The listing builds one solid part. Answer for the finished solid, in the listing's coordinates (mm). A direction names the side the tool comes from. Give positions to 0.01 mm unless a question says otherwise; leave off trailing zeros. Loops run counter-clockwise (first coordinate to the right, second up) from the corner with the lowest first, then second, coordinate; pieces in that order, holes last. Notation, with made-up numbers: M -35.75,15 L -25.75,15 A26 ccw -25.75,41 Z; hole C 78.25,-17 d2. An arc over 180 degrees is marked long. Return JSON: item names as keys, results as strings.
Autodesk Inventor part; units mm, degrees
ref_plane "YZ Plane" through (0, 0, 0) normal (1, 0, 0) x (0, 1, 0)
ref_plane "XZ Plane" through (0, 0, 0) normal (0, 1, 0) x (-1, 0, 0)
ref_plane "XY Plane" through (0, 0, 0) normal (0, 0, 1) x (1, 0, 0)
sketch "Эскиз1" plane through (0, 0, 0) normal (0, 0, 1) x (1, 0, 0)
  line L0 (0, 5) -> (0, 0)
  line L1 (0, 0) -> (36, 0)
  line L2 (36, 0) -> (36, 10)
  line L3 (36, 10) -> (16, 10)
  line L4 (16, 10) -> (16, 5)
  line L5 (16, 5) -> (0, 5)
  dimension "d0" = 5
  dimension "d1" = 20
  dimension "d3" = 10
  dimension "d4" = 36
revolve "Вращение1" add sketch "Эскиз1" angle 360 about axis through (0, 5, 0) along (0, -1, 0)
sketch "Эскиз2" plane through (0, 0, 0) normal (1, 0, 0) x (0, 1, 0)
  line L0 (-2, 0) -> (12, 0)
  line L1 (0, -34) -> (0, 64)
  line L2 (0, 0) -> (0, 50)
  line L3 (0, 50) -> (10, 50)
  line L4 (10, 50) -> (10, 0)
  line L5 (0, 0) -> (10, 0)
  line L6 (10, 36) -> (0, 36)
  dimension "d6" = 10
  dimension "d7" = 50
revolve "Вращение2" add sketch "Эскиз2" angle 360 about axis through (0, -10, 0) along (0, 1, 0)
chamfer "Фаска1" distance 1 angle 45 1 edges at (0, 0, -50)
sketch "Эскиз3" plane through (0, 0, 0) normal (0, -1, 0) x (1, 0, 0)
  circle A0 centre (0, 0) radius 42.5 construction
  circle A1 centre (0, 42.5) radius 5.5
  line L0 (0, -70) -> (0, 70)
  line L1 (-70, 0) -> (70, 0)
  dimension "d10" = 85
  dimension "d9" = 11
hole "Отверстие1" at (0, 0, 42.5) direction (0, 1, 0) diameter 6.2 depth 15 tip angle 118 counterbore diameter 11 counterbore depth 6.8
pattern_circular "Круговой массив1" count 6 over 360 about axis through (0, -10, 0) along (0, 1, 0) of "Отверстие1"
sketch "Эскиз4" plane through (0, 10, 0) normal (0, 1, 0) x (1, 0, 0)
  circle A0 centre (0, 0) radius 36
  circle A1 centre (0, 0) radius 16
  circle A2 centre (0, 0) radius 16
  circle A3 centre (0, 0) radius 36
  dimension "d27" = 72
extrude "Выдавливание2" add sketch "Эскиз4" along normal blind 8
fillet "Сопряжение1" radius 1.3 1 edges at (-36, 10, 0)
sketch "Эскиз5" plane through (0, 0, 0) normal (0, -1, 0) x (1, 0, 0)
  line L0 (-70, 0) -> (70, 0)
  line L1 (0, 70) -> (0, -70)
  circle A0 centre (0, 0) radius 21
  dimension "d31" = 42
extrude "Выдавливание3" cut sketch "Эскиз5" against normal blind 50
chamfer "Фаска2" distance 1 angle 45 2 edges at (-21, 0, 0) (-21, 18, 0)
chamfer "Фаска3" distance 2 angle 45 1 edges at (-36, 18, 0)
properties part number "Крышка большая_ПОД МАНЖЕТУ"
(1) Given pin 1 (9 mm diameter, centred on x = 0, z = -42.5, fed in from -Y); pin 2 (10 mm diameter, centred on x = 0, z = 42.5, fed in from +Y); pin 3 (14.5 mm diameter, centred on x = 36.81, z = -21.25, fed in from +Y); pin 4 (5.5 mm diameter, centred on x = 36.81, z = -21.25, fed in from -Y), each flat-ended and moving along its own axis, determine where each tip first touches the part or whether it passes through.
Values follow:
{"pin 1": "y = 6.8", "pin 2": "y = 10", "pin 3": "y = 16.75", "pin 4": "through"}
(2) The part is cut by section B-B (y = 14.75). Determine the outline of the cut face in (x, z).
Values follow:
{"outline": "C 0,0 d72; hole C 0,0 d42"}
(3) Straight lines are drawn through the part: line 1 along X through (y, z) = (11.25, 0); line 2 along X through (y, z) = (7.9, -21.25); line 3 along X through (y, z) = (4.75, 0). For each, find the intervals that lie inside material, in ascending order.
Values follow:
{"line 1": "-36 to -21, 21 to 36", "line 2": "-45.26 to -39.91, -33.71 to 33.71, 39.91 to 45.26", "line 3": "-50 to -21, 21 to 50"}
(4) Determine the mould class of faces 3 (the cylindrical face through (15.02, 5.56, 47.69)), 4 (the cylindrical face through (-42.175, 3.448, 20.058)), 5 (the flat face through (-10, 0, 21)) for opening direction Z: released by +Z, released by -Z, zero draft, split by the parting line, or undercut.
Values follow:
{"face 3": "split by the parting line", "face 4": "undercut", "face 5": "zero draft"}
(5) The part is cut by section C-C (x = 0). Give the number of separate pieces and of enclosed holes in the cut face, and give its area (3 significant figures).
Values follow:
{"separate pieces": "4", "enclosed holes": "0", "area": "624 mm²"}
(6) A tool of negligible diameter and unlimited length cuts with its end or side. For faces 1 (the flat face through (2.4, 6.8, 40.1)), 2 (the cylindrical face through (1.187, 8.422, 39.636)), from which of +Z, -Z, +X, -X, +Y, -Y can it reach the whole face along a straight path? Write none if from no direction.
Values follow:
{"face 1": "-Y", "face 2": "+Y, -Y"}
(7) The part is cut by section D-D (y = 4.75). Determine the outline of the cut face in (x, z).
Values follow:
{"outline": "C 0,0 d100; hole C -36.81,-21.25 d11; hole C -36.81,21.25 d11; hole C 0,0 d42; hole C 0,-42.5 d11; hole C 0,42.5 d11; hole C 36.81,-21.25 d11; hole C 36.81,21.25 d11"}
(8) The part is cut by section A-A (z = 0). Determine the outline of the cut face in (x, y), and give its area (3 significant figures).
Values follow:
{"outline": "M -50,1 L -49,0 L -22,0 L -21,1 L -21,17 L -22,18 L -34,18 L -36,16 L -36,11.3 A1.3 cw -37.3,10 L -50,10 Z; M 21,1 L 22,0 L 49,0 L 50,1 L 50,10 L 37.3,10 A1.3 cw 36,11.3 L 36,16 L 34,18 L 22,18 L 21,17 Z", "area": "814 mm²"}
